Autodesk Inventor part; units mm, degrees
ref_plane "YZ Plane" through (0, 0, 0) normal (1, 0, 0) x (0, 1, 0)
ref_plane "XZ Plane" through (0, 0, 0) normal (0, 1, 0) x (-1, 0, 0)
ref_plane "XY Plane" through (0, 0, 0) normal (0, 0, 1) x (1, 0, 0)
sketch "Sketch1" plane through (0, 0, 0) normal (0, 0, 1) x (1, 0, 0)
  circle A0 centre (0, 0) radius 1.7145
  arc A1 (-1.687, 3.0581) -> (3.0246, -1.7462) centre (0, 0) ccw
  circle A2 centre (36.2951, -20.955) radius 1.7145
  arc A3 (33.5455, -19.3675) -> (39.4701, -20.955) centre (36.2951, -20.955) ccw
  line L0 (0, 0) -> (44.3838, 0) construction
  arc A4 (39.4701, -16.6464) -> (6.2054, 4.5403) centre (0, -41.91) ccw
  line L1 (33.1201, -20.955) -> (33.1201, -12.2644)
  line L2 (39.4701, -20.955) -> (39.4701, -16.6464)
  arc A5 (6.2054, 4.5403) -> (-1.687, 3.0581) centre (4.5073, -8.1706) ccw
  line L3 (0, 0) -> (36.2951, -20.955) construction
  line L4 (3.0246, -1.7462) -> (-1.8014, -10.1051)
  line L5 (-1.8014, -10.1051) -> (12.1007, -18.1315)
  line L6 (12.1007, -18.1315) -> (16.9267, -9.7726)
  line L7 (16.9267, -9.7726) -> (20.993, -2.7297)
  arc A6 (33.1201, -12.2644) -> (20.993, -2.7297) centre (0, -41.91) ccw
  dimension "d0" = 3.429
  dimension "d1" = 6.985
  dimension "d2" = 3.429
  dimension "d3" = 6.35
  dimension "d4" = 30
  dimension "d5" = 41.91
  dimension "d6" = 93.726
  dimension "d7" = 41.91
  dimension "d10" = 16.0528
  dimension "d11" = 9.652
extrude "Extrusion1" add sketch "Sketch1" along normal blind 3.81
fillet "Fillet1" radius 3.175 4 edges at (3.0246, -1.7462, 1.905) (20.993, -2.7297, 1.905) (33.1201, -12.2644, 1.905) (39.4701, -16.6464, 1.905)
sketch "Sketch2" plane through (0, 0, 3.81) normal (0, 0, 1) x (1, 0, 0)
  line L0 (-1.8014, -10.1051) -> (12.1007, -18.1315)
  line L1 (12.1007, -18.1315) -> (9.901, -16.8615)
  line L2 (14.727, -8.5026) -> (16.9267, -9.7726)
  line L3 (12.1007, -18.1315) -> (19.3978, -5.4927)
  line L4 (12.1007, -18.1315) -> (16.9267, -9.7726)
  line L5 (-0.3054, -7.5139) -> (-1.8014, -10.1051)
  line L6 (-1.8014, -10.1051) -> (3.0246, -1.7463)
  line L7 (3.0246, -1.7463) -> (5.2243, -3.0163)
  line L8 (0.3983, -11.3751) -> (-1.8014, -10.1051)
  line L9 (11.171, -14.6618) -> (12.0509, -15.1698)
  line L10 (12.0509, -15.1698) -> (11.5429, -16.0497)
  line L11 (11.5429, -16.0497) -> (10.663, -15.5417)
  line L12 (1.6683, -9.1754) -> (0.7884, -8.6674)
  line L13 (0.7884, -8.6674) -> (0.2804, -9.5473)
  line L14 (0.2804, -9.5473) -> (1.1603, -10.0553)
  line L15 (5.2243, -3.0163) -> (1.6683, -9.1754)
  line L16 (1.1603, -10.0553) -> (0.3983, -11.3751)
  line L17 (9.901, -16.8615) -> (10.663, -15.5417)
  line L18 (11.171, -14.6618) -> (14.727, -8.5026)
  point P0 (0, 0)
  dimension "d15" = 9.652
  dimension "d17" = 2.54
  dimension "d18" = 7.112
  dimension "d19" = 7.112
  dimension "d20" = 1.016
  dimension "d21" = 1.016
extrude "Extrusion2" add sketch "Sketch2" along normal blind 4.318
properties part number "BatteryBalanceConnectorHolder"
Source: CAD feature listing. Evaluate the final solid. Frame: model axes, mm. A direction names the side the tool comes from. Coordinates: 2 decimals unless noted, no trailing zeros. Loops run counter-clockwise (first coordinate to the right, second up) from the corner with the lowest first, then second, coordinate; pieces in that order, holes last. Notation, with made-up numbers: (3, -13.5) - (38, -13.5) arc R36 cw to (38, 22.5) - close; hole circle Ø8 at (-6, -6). An arc over 180 degrees is marked (long way). One line per item, written item: value. Start each with the question number.
1. Section A-A (z = 5.5). Return the cut outline in (x, y).
2. Mould query, pull axis X, two halves, no side actions, for faces 4 (the flat face through (11.11, -15.8, 5.94)), 5 (the flat face through (15.81, -9.13, 5.94)), 6 (the flat face through (10.277, -16.211, 5.939)). Classes: pulls with the +X half, pulls with the -X half, needs draft (parallel to the pull), parting line crosses it, or undercut.
3. Section B-B (y = -20.25). Return the cut outline in (x, z).
4. Section C-C (y = 0). Return the cut outline in (x, z), and give its area (3 significant figures).
5. Set-up query: faces 1 (the flat face through (11.8, -15.604, 5.939)), 2 (the cylindrical face through (32.9, -12.34, 1.93)), 3 (the flat face through (0.78, -10.71, 5.94)). Return all of +Z, -Z, +X, -X, +Y, -Y with unobstructed straight access to the full face (end or side cutting, diameter ignored); none if empty.
6. Section D-D (x = 31). Return the cut outline in (y, z), and give its area (3 significant figures).
7. Contact query for flat-ended pins moving along their axis: P1, Ø3, axis at x = 31.5, z = 1.5, coming from the +Y side; P2, Ø1.1, axis at y = -16, z = 2, coming from the -X side; P3, Ø1, axis at x = 1.5, y = -2, coming from the +Z side; P4, Ø2, axis at x = 36.3, y = -20.96, coming from the -Z side. Output: stop coordinate, or through.
8. Ray query, L1, parallel to Z at x = 5.5, y = 0.25; L2, parallel to X at y = -1.5, z = 2.5; L3, parallel to X at y = -1, z = 3. Return the intervals inside material, ascending.
Verdict:
1. outline: (-1.8, -10.11) - (0.4, -11.38) - (1.16, -10.06) - (0.28, -9.55) - (0.79, -8.67) - (1.67, -9.18) - (5.22, -3.02) - (3.02, -1.75) - (-0.31, -7.51) - close; (9.9, -16.86) - (12.1, -18.13) - (16.93, -9.77) - (14.73, -8.5) - (11.17, -14.66) - (12.05, -15.17) - (11.54, -16.05) - (10.66, -15.54) - close
2. face 4: undercut
2. face 5: pulls with the +X half
2. face 6: pulls with the -X half
3. outline: (33.12, 0) - (34.73, 0) - (34.73, 3.81) - (33.12, 3.81) - close; (37.86, 0) - (39.47, 0) - (39.47, 3.81) - (37.86, 3.81) - close
4. outline: (-3.49, 0) - (-1.71, 0) - (-1.71, 3.81) - (-3.49, 3.81) - close; (1.71, 0) - (20.97, 0) - (20.97, 3.81) - (1.71, 3.81) - close
4. area: 80.1 mm2
5. face 1: +Z
5. face 2: +Z, -Z, -Y
5. face 3: +Z, -Y
6. outline: (-10.05, 0) - (-6.77, 0) - (-6.77, 3.81) - (-10.05, 3.81) - close
6. area: 12.5 mm2
7. P1: stops at y = -5.91
7. P2: stops at x = 7.46
7. P3: stops at z = 3.81
7. P4: passes through
8. L1: z = 0 to 3.81
8. L2: x = -3.15 to -0.83, 0.83 to 23.73
8. L3: x = -3.35 to -1.39, 1.39 to 22.86
